```python
from build123d import *

# Parameters (mm, degrees)
F2_DEPTH = 20
F3_DEPTH = 56
F4_DEPTH = 52


with BuildPart() as f2:
    # F0 (on Top) → F2 (new body)
    with BuildSketch(Plane.XY):
        with BuildLine():
            Line((200, 0), (0, 0))
            Line((0, 0), (0, -14.61))
            ThreePointArc((0, -14.61), (13.843459, -27.728929), (32.309226, -32.5))
            Line((32.309226, -32.5), (32.309226, -14.61))
            Line((32.309226, -14.61), (69.309226, -14.61))
            Line((69.309226, -14.61), (69.309226, -32.5))
            Line((69.309226, -32.5), (107.261054, -32.5))
            ThreePointArc((107.261054, -32.5), (113.322375, -25.56096), (115.506455, -16.61))
            Line((115.506455, -16.61), (115.506455, -14.61))
            Line((115.506455, -14.61), (154.339641, -14.61))
            ThreePointArc((154.339641, -14.61), (177.560637, -14.834695), (200, -8.85639))
            Line((200, -8.85639), (200, 0))
        make_face()
    extrude(amount=-F2_DEPTH)

    # F1 (on Right) → F3 (join)
    with BuildSketch(Plane.YZ):
        with BuildLine():
            Line((0, -38.5), (0, -19.5))
            ThreePointArc((0, -19.5), (-9.5, -29), (0, -38.5))
        make_face()
        with BuildLine():
            Line((0, -19.5), (0, -11.71401))
            Line((0, -11.71401), (-13.5, -11.71401))
            Line((-13.5, -11.71401), (-13.5, -29))
            ThreePointArc((-13.5, -29), (-9.545942, -38.545942), (0, -42.5))
            Line((0, -42.5), (0, -38.5))
            ThreePointArc((0, -38.5), (-9.5, -29), (0, -19.5))
        make_face()
    extrude(amount=F3_DEPTH)

    # F1 (on Right) → F4 (cut)
    with BuildSketch(Plane.YZ):
        with BuildLine():
            Line((0, -38.5), (0, -19.5))
            ThreePointArc((0, -19.5), (-9.5, -29), (0, -38.5))
        make_face()
    extrude(amount=-F4_DEPTH, mode=Mode.SUBTRACT)


solid = f2.part
```
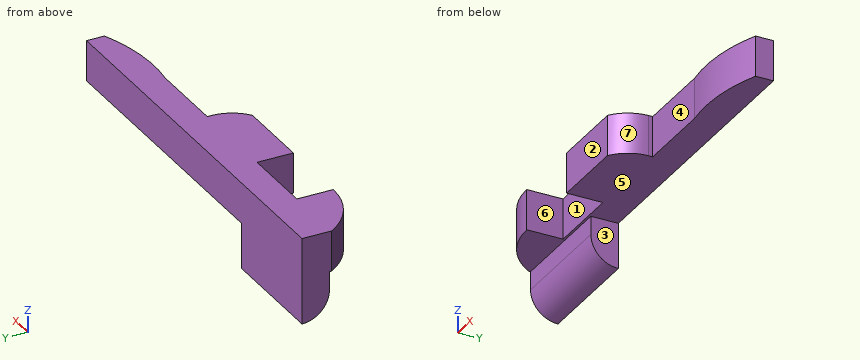
CAD build for the part. Positions are in the model's coordinates, mm. Face numbers are marked on the shaded views. A direction names the side the tool comes from. Give positions to 0.01 mm unless a question says otherwise; leave off trailing zeros. Order: outer loops, then holes, each group sorted by start corner. A loop starts at its lowest first (then second) coordinate and runs counter-clockwise, first axis right, second up. Notation, with made-up numbers: M -39.75,14.5 L 17.25,14.5 A21 ccw 17.25,34.5 Z; hole C -36,-19.75 d1. An arc over 180 degrees is marked long. Put each result on its own line as item: value. Start each with the question number.
(1) Flat gauge pins, fed straight in: pin 1 Ø4.5 at (x, z) = (40.5, -23) entering from -Y; pin 2 Ø22 at (x, z) = (127, -6) entering from -Y; pin 3 Ø6 at (x, z) = (92, -22) entering from +Y; pin 4 Ø9 at (y, z) = (-25, -12.5) entering from +X. Where does each tip first touch, or does it go through?
(2) Saw through at A-A, the plane y = -22.5. Write the cut outline in (x, z), then the cut area to 3 significant figures.
(3) Drill centre lines: line 1 along Z through (x, y) = (175.5, -15); line 2 along Y through (x, z) = (153, -5.5); line 3 along Y through (x, z) = (44, -26.5). Where is each one in solid material? Low to high.
(4) Which spindle directions (+Z, -Z, +X, -X, +Y, -Y) get a long thin tool onto all of the face, cutting with end or side? Do the marked faces 1, 2 and 3. Say none if no direction does.
(5) Mould opens along X. For the marked faces 4, 5, 6 and 7 say: +X half, -X half, draft (parallel to the pull), parting line (faces both ways), or undercut.
(6) Saw through at D-D, the plane x = 148. Write the cut outline in (y, z), then the cut area to 3 significant figures.
(7) Saw through at C-C, the plane z = -5. Write the cut outline in (x, y).
(8) Saw through at B-B, the plane x = 53. Write the cut outline in (y, z), then the cut area to 3 significant figures.
Check result:
1. pin 1: stops at y = -13.5
1. pin 2: stops at y = -14.61
1. pin 3: stops at y = 0
1. pin 4: stops at x = 115.11
2. outline: M 6.57,-20 L 32.31,-20 L 32.31,0 L 6.57,0 Z; M 69.31,-20 L 114.59,-20 L 114.59,0 L 69.31,0 Z
2. area: 1,420 mm2
3. line 1: z = -20 to 0
3. line 2: y = -14.61 to 0
3. line 3: y = -13.5 to 0
4. face 1: +Z, -Z, -Y
4. face 2: +Z, -Z, +X, -X, -Y
4. face 3: -Z, +X, +Y, -Y
5. face 4: undercut
5. face 5: draft
5. face 6: undercut
5. face 7: +X half
6. outline: M -14.61,-20 L 0,-20 L 0,0 L -14.61,0 Z
6. area: 292 mm2
7. outline: M 0,-14.61 A38.12 ccw 32.31,-32.5 L 32.31,-14.61 L 69.31,-14.61 L 69.31,-32.5 L 107.26,-32.5 A19.43 ccw 115.51,-16.61 L 115.51,-14.61 L 154.34,-14.61 A86.25 ccw 200,-8.86 L 200,0 L 0,0 Z
8. outline: M -14.61,-20 L -13.5,-20 L -13.5,-29 A13.5 ccw 0,-42.5 L 0,0 L -14.61,0 Z
8. area: 557 mm2
